Verification items for the finished model (mm, model axes). A direction names the side the tool comes from. Give positions to 0.01 mm unless a question says otherwise; leave off trailing zeros. Loops run counter-clockwise (first coordinate to the right, second up) from the corner with the lowest first, then second, coordinate; pieces in that order, holes last. Notation, with made-up numbers: M 25.5,-21.75 L 54.5,-21.75 A22 ccw 54.5,4.25 Z; hole C 46.25,-13.5 d8. An arc over 180 degrees is marked long. Use a Markdown table: item, result.
from build123d import *

# Parameters (mm, degrees)
SKETCH1_R           = 2
BOSS_EXTRUDE1_DEPTH = 24
SKETCH3_R           = 3
BOSS_EXTRUDE3_DEPTH = 9
BOSS_EXTRUDE4_START = 14
SKETCH4_R           = 2
BOSS_EXTRUDE4_DEPTH = 14
CUT_EXTRUDE1_START  = -3
SKETCH5_R           = 4
SKETCH5_R_2         = 2
CUT_EXTRUDE1_DEPTH  = 3


with BuildPart() as part:
    # Sketch1 → Boss-Extrude1 (new body)
    with BuildSketch(Plane.XY):
        Circle(SKETCH1_R)
    extrude(amount=BOSS_EXTRUDE1_DEPTH)

    # Sketch3 → Boss-Extrude3 (add)
    with BuildSketch(Plane.XY.offset(19)):
        Circle(SKETCH3_R)
    extrude(amount=-BOSS_EXTRUDE3_DEPTH)

    # Sketch4 → Boss-Extrude4 (add)
    with BuildSketch(Plane(origin=(0, 0, 0), x_dir=(-1, 0, 0), z_dir=(0, 0, -1)).offset(BOSS_EXTRUDE4_START)):
        Circle(SKETCH4_R)
    extrude(amount=-BOSS_EXTRUDE4_DEPTH)

    # Sketch5 → Cut-Extrude1 (cut)
    with BuildSketch(Plane.XY.offset(19).offset(CUT_EXTRUDE1_START)):
        Circle(SKETCH5_R)
        with Locations(Location((0, 0, 0), (0, 0, 180))):
            Circle(SKETCH5_R_2, mode=Mode.SUBTRACT)
    extrude(amount=CUT_EXTRUDE1_DEPTH, mode=Mode.SUBTRACT)


solid = part.part
(1) Cross-section at A-A on x = 0. Record the cut outline in (y, z), then the cut area to 3 significant figures.
Results below:
| item | result |
|---|---|
| outline | M -3,10 L -2,10 L -2,-14 L 2,-14 L 2,10 L 3,10 L 3,16 L 2,16 L 2,24 L -2,24 L -2,16 L -3,16 Z |
| area | 164 mm^2 |
(2) Cross-section at D-D on z = 1.5. Record the cut outline in (x, y).
Results below:
| item | result |
|---|---|
| outline | C 0,0 d4 |
(3) Cross-section at C-C on z = 12. Record the cut outline in (x, y).
Results below:
| item | result |
|---|---|
| outline | C 0,0 d6 |
(4) Material ranges on line 1 (Z direction, x = -1.95, y = 1.05); line 2 (X direction, y = 0, z = 7.5); line 3 (Y direction, x = 1.05, z = 0.5), recorded low to high.
Results below:
| item | result |
|---|---|
| line 1 | 10 to 16 |
| line 2 | -2 to 2 |
| line 3 | -1.7 to 1.7 |
(5) Gauge pin test, flat end, axial feed: P1, Ø3, axis at x = 1.5, z = 6.5, coming from the +Y side. Record the tip position at first contact, or that the pin passes through.
Results below:
| item | result |
|---|---|
| P1 | y = 2 |
(6) Set-up check for faces 1 (the flat face through (1, -2, 10)), 2 (the flat face through (0, 0, 24)), 3 (the flat face through (1, -2, 16)): record each of +Z, -Z, +X, -X, +Y, -Y from which the full face is reachable in a straight line by a thin tool's end or side.
Results below:
| item | result |
|---|---|
| face 1 | -Z |
| face 2 | +Z, +X, -X, +Y, -Y |
| face 3 | +Z |
